Work out the finished part from the listing and answer in its coordinate system (mm). A direction names the side the tool comes from. Coordinates: 2 decimals unless noted, no trailing zeros. Order: outer loops, then holes, each group sorted by start corner. A loop starts at its lowest first (then second) coordinate and runs counter-clockwise, first axis right, second up. Notation, with made-up numbers: (23, -34) -> (55, -34) arc R28 cw to (55, 2) -> close; hole circle Ø1 at (4, 68.25). An arc over 180 degrees is marked (long way). Write item = value, one per line. Start each with the question number.
Q1. The part is cut by section A-A, the plane y = -64. Determine the outline of the cut face in (x, z).
Q2. Straight lines are drawn through the part: L1, parallel to Y at x = 3.5, z = 9.5; L2, parallel to Z at x = -6.25, y = -38.5; L3, parallel to Y at x = -8.5, z = -5. For each, find the intervals that lie inside material, in ascending order. Write a range as from..to.
Q3. Flat-ended cylindrical pins translate along their axes: pin 1 (5 mm diameter, centred on y = -33.5, z = 4, fed in from +X); pin 2 (6 mm diameter, centred on y = -29.5, z = -7.5, fed in from -X); pin 3 (2 mm diameter, centred on y = -53, z = 0, fed in from -X). Find the tip coordinate at first contact, or state that the pin passes through.
Q4. Which of the six approach directions +Z, -Z, +X, -X, +Y, -Y give full straight-line access (tool end or side, diameter ignored) to faces 1 (the cylindrical face through (-2.17, -36.48, -9.76)), 2 (the conical face through (-12.598, 11.696, -7.232))?
```python
from build123d import *

# Parameters (mm, degrees)
BOSS_EXTRUDE1_DEPTH = 12
SKETCH2_OUTSIDE_W   = 80.454
SKETCH2_OUTSIDE_H   = 84.786
SKETCH2_OUTSIDE_R   = 14
CUT_EXTRUDE1_DEPTH  = 12
CUT_EXTRUDE1_TAPER  = 60
SKETCH3_R           = 10
BOSS_EXTRUDE2_DEPTH = 75
CHAMFER1_SIZE       = 1


with BuildPart() as part:
    # Sketch1 → Boss-Extrude1 (new body)
    with BuildSketch(Plane(origin=(0, 0, 0), x_dir=(1, 0, 0), z_dir=(0, 1, 0))):
        Polygon((0, -16.165807537), (14, -8.082903769), (14, 8.082903769), (0, 16.165807537), (-14, 8.082903769), (-14, -8.082903769), align=None)
    extrude(amount=BOSS_EXTRUDE1_DEPTH)

    # Sketch2 outside → Cut-Extrude1 (cut)
    with BuildSketch(Plane(origin=(0, 12, 0), x_dir=(1, 0, 0), z_dir=(0, 1, 0))):
        Rectangle(SKETCH2_OUTSIDE_W, SKETCH2_OUTSIDE_H)
        Circle(SKETCH2_OUTSIDE_R, mode=Mode.SUBTRACT)
    extrude(amount=-CUT_EXTRUDE1_DEPTH, taper=CUT_EXTRUDE1_TAPER, mode=Mode.SUBTRACT)

    # Sketch3 → Boss-Extrude2 (add)
    with BuildSketch(Plane.XZ):
        Circle(SKETCH3_R)
    extrude(amount=BOSS_EXTRUDE2_DEPTH)

    # Chamfer1
    chamfer1_edges = [part.edges().sort_by_distance(p)[0] for p in [
        (-10, -75, 0),
    ]]
    chamfer(chamfer1_edges, length=CHAMFER1_SIZE)


solid = part.part
```
Model answer:
q1.outline = circle Ø20 at (0, 0)
q2.L1 = 0..12
q2.L2 = -7.81..7.81
q2.L3 = -74.14..12
q3.pin_1 = 9.89
q3.pin_2 = -8.93
q3.pin_3 = -10
q4.face_1 = -Y
q4.face_2 = -Z, -X, +Y
